CAD build for the part. Positions are in the model's coordinates, mm. Round coordinates to 2 decimals unless told otherwise and drop trailing zeros. Write each loop counter-clockwise with the first axis right and the second up, starting at its lowest first coordinate (ties: lowest second). Pieces come first, ordered by that corner, then holes. Notation, with made-up numbers: (39.25, 45) - (43.25, 45) arc R23 cw to (43.25, 75) - close; hole circle Ø2 at (-11.75, -6). An arc over 180 degrees is marked (long way). Put each result on its own line as item: value. Start each with the question number.
Item 1: Pin check, flat tips, straight feed: pin 1 Ø4 at (x, y) = (67.5, 52.5) entering from -Z; pin 2 Ø3 at (x, y) = (-78.83, 51.98) entering from -Z. Stop position of each tip, or through.
Item 2: Cut at B-B (y = 74.84). Give the cut face in (x, z).
Item 3: Cut at A-A (x = -58.3). Give the cut face in (y, z).
Item 4: Drill centre lines: line 1 (Y direction, x = 78.65, z = 1.2); line 2 (Y direction, x = -78.83, z = 0.35). Where is each one in solid material? Low to high. Write a range as from..to.
Item 5: Mould opens along Y. For faces 1 (the cylindrical face through (28.7, 24.6, 0.8)), 2 (the cylindrical face through (84, 83, 1)), 3 (the flat face through (-1, 1, 0)) say: released by +Y, released by -Y, zero draft, split by the parting line, or undercut.
```python
from build123d import *

# Parameters (mm, degrees)
SKETCH1_W            = 170
SKETCH1_H            = 170
BASE_DEPTH           = 1.6
ROUNDING_CORNERS_R   = 5
SKETCH2_R            = 2.03
MOUNTING_HOLES_DEPTH = 1.6
SKETCH4_R            = 3
COOLER_HOLES_DEPTH   = 1.6


with BuildPart() as part:
    # Sketch1 → Base (new body)
    with BuildSketch(Plane.XY):
        Rectangle(SKETCH1_W, SKETCH1_H)
    extrude(amount=BASE_DEPTH)

    # Rounding corners
    rounding_corners_edges = [part.edges().sort_by_distance(p)[0] for p in [
        (-85, 85, 0.8),
        (85, 85, 0.8),
        (85, -85, 0.8),
        (-85, -85, 0.8),
    ]]
    fillet(rounding_corners_edges, radius=ROUNDING_CORNERS_R)

    # Sketch2 → Mounting holes (cut)
    with BuildSketch(Plane.XY.offset(1.6)):
        with Locations((-78.83, 51.98)):
            Circle(SKETCH2_R)
        with Locations((78.65, 74.84)):
            Circle(SKETCH2_R)
        with Locations((-78.83, -80.1)):
            Circle(SKETCH2_R)
        with Locations((78.65, -80.1)):
            Circle(SKETCH2_R)
    extrude(amount=-MOUNTING_HOLES_DEPTH, mode=Mode.SUBTRACT)

    # Sketch4 → Cooler holes (cut)
    with BuildSketch(Plane.XY.offset(1.6)):
        with Locations((-58.3, 24.5)):
            Circle(SKETCH4_R)
        with Locations((31.7, 24.5)):
            Circle(SKETCH4_R)
        with Locations((31.7, -29.5)):
            Circle(SKETCH4_R)
        with Locations((-58.3, -29.5)):
            Circle(SKETCH4_R)
    extrude(amount=-COOLER_HOLES_DEPTH, mode=Mode.SUBTRACT)


solid = part.part
```
Output values:
1. pin 1: z = 0
1. pin 2: through
2. outline: (-85, 0) - (76.62, 0) - (76.62, 1.6) - (-85, 1.6) - close; (80.68, 0) - (85, 0) - (85, 1.6) - (80.68, 1.6) - close
3. outline: (-85, 0) - (-32.5, 0) - (-32.5, 1.6) - (-85, 1.6) - close; (-26.5, 0) - (21.5, 0) - (21.5, 1.6) - (-26.5, 1.6) - close; (27.5, 0) - (85, 0) - (85, 1.6) - (27.5, 1.6) - close
4. line 1: -85..-82.13, -78.07..72.81, 76.87..85
4. line 2: -85..-82.13, -78.07..49.95, 54.01..85
5. face 1: undercut
5. face 2: released by +Y
5. face 3: zero draft
